Read the model definition and answer for the solid it produces. Units are mm, in the model's axes. Face numbers are marked on the shaded views. A direction names the side the tool comes from. Give positions to 0.01 mm unless a question says otherwise; leave off trailing zeros. Order: outer loops, then holes, each group sorted by start corner. A loop starts at its lowest first (then second) coordinate and runs counter-clockwise, first axis right, second up.
```python
from build123d import *

# Parameters (mm, degrees)
F0_R     = 6.375
F1_DEPTH = 8.26
F0_R_2   = 9.525
F2_DEPTH = 14.26
F3_W     = 13.49
F3_H     = 58.49083
F4_DEPTH = 38


with BuildPart() as f1:
    # F0 (on Front) → F1 (new body, symmetric)
    with BuildSketch(Plane.XZ):
        with BuildLine():
            Line((-26.615233, 45.963348), (-25.360972, 33.179498))
            ThreePointArc((-25.360972, 33.179498), (-9.404585, 28.615193), (4.051067, 38.330365))
            Line((4.051067, 38.330365), (10.939452, 38.330365))
            ThreePointArc((10.939452, 38.330365), (4.770442, 45.680142), (-0.28538, 53.835787))
            ThreePointArc((-0.28538, 53.835787), (-16.692609, 60.743646), (-26.615233, 45.963348))
        make_face()
        with Locations((-12.682133, 47.330365)):
            Circle(F0_R, mode=Mode.SUBTRACT)
    extrude(amount=F1_DEPTH, both=True)

    # F0 (on Front) → F2 (join, symmetric)
    with BuildSketch(Plane.XZ):
        with BuildLine():
            Line((-25.360972, 33.179498), (-21.894871, -2.14817))
            ThreePointArc((-21.894871, -2.14817), (-14.189314, -16.812596), (1.561379, -21.944523))
            Line((1.561379, -21.944523), (57, -18))
            Line((57, -18), (57, -6.375))
            Line((57, -6.375), (35, -6.375))
            ThreePointArc((35, -6.375), (28.625, 0), (35, 6.375))
            Line((35, 6.375), (57, 6.375))
            Line((57, 6.375), (57, 18))
            ThreePointArc((57, 18), (31.987423, 23.674071), (10.939452, 38.330365))
            Line((10.939452, 38.330365), (4.051067, 38.330365))
            ThreePointArc((4.051067, 38.330365), (-9.404585, 28.615193), (-25.360972, 33.179498))
        make_face()
        Circle(F0_R_2, mode=Mode.SUBTRACT)
    extrude(amount=F2_DEPTH, both=True)

    # F3 (on face) → F4 (cut)
    with BuildSketch(Plane.YZ.offset(57)):
        with Locations((0, -0.116389)):
            Rectangle(F3_W, F3_H)
    extrude(amount=-F4_DEPTH, mode=Mode.SUBTRACT)


solid = f1.part
```
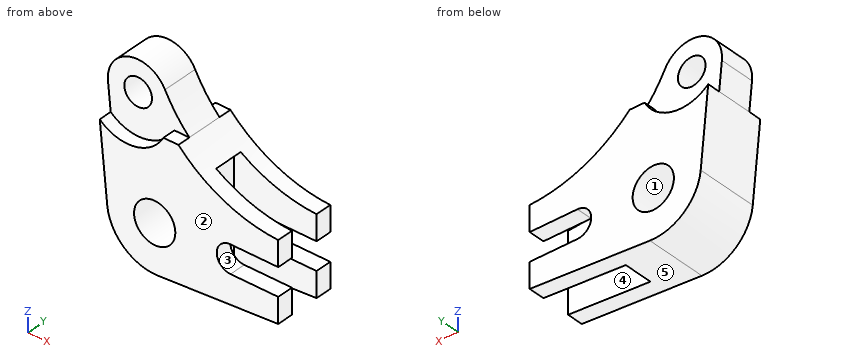
1) The part is cut by section D-D on z = 31.5. Determine the outline of the cut face in (x, y), and give its area (3 significant figures).
Final values:
outline: (-25.2, -14.26) - (-23.19, -14.26) - (-23.19, -8.26) - (-2.18, -8.26) - (-2.18, -14.26) - (18.67, -14.26) - (18.67, 14.26) - (-2.18, 14.26) - (-2.18, 8.26) - (-23.19, 8.26) - (-23.19, 14.26) - (-25.2, 14.26) - close
area: 999 mm2
2) A tool of negligible diameter and unlimited length cuts with its end or side. For the marked faces 4 and 5, from which of +Z, -Z, +X, -X, +Y, -Y can it reach the whole face along a straight path? Write none if from no direction.
Final values:
face 4: -Z, +X
face 5: -Z, +X, +Y, -Y
3) Consider L1, parallel to Y at x = 31.5, z = 6 (3 decimals); L2, parallel to Z at x = 0, y = -9.25 (3 decimals); L3, parallel to X at y = 10, z = 6.5. Determine where each line is inside the solid, lowest interval first.
Final values:
L1: y = -14.26 to -6.745, 6.745 to 14.26
L2: z = -22 to -9.525, 9.525 to 33.182
L3: x = -22.74 to -6.96, 6.96 to 57
4) Given pin 1 (6 mm diameter, centred on y = 4, z = 32, fed in from -X); pin 2 (8 mm diameter, centred on y = -10.5, z = 39, fed in from +X); pin 3 (5 mm diameter, centred on x = 7, y = -11, fed in from +Z), each flat-ended and moving along its own axis, determine where each tip first touches the part or whether it passes through.
Final values:
pin 1: stops at x = -25.54
pin 2: stops at x = 14.41
pin 3: stops at z = 38.33
5) The part is cut by section A-A on z = 0. Determine the outline of the cut face in (x, y) (3 decimals), and give its area (3 significant figures).
Final values:
outline: (-22.106, -14.26) - (-9.525, -14.26) - (-9.525, 14.26) - (-22.106, 14.26) - close; (9.525, -14.26) - (28.625, -14.26) - (28.625, -6.745) - (19, -6.745) - (19, 6.745) - (28.625, 6.745) - (28.625, 14.26) - (9.525, 14.26) - close
area: 774 mm2
6) The part is cut by section C-C on y = 2. Count the separate pieces of the cut face and the enclosed holes in it, and give its area (3 significant figures).
Final values:
separate pieces: 1
enclosed holes: 2
area: 2,610 mm2
7) The part is cut by section B-B on x = 51. Determine the outline of the cut face in (y, z) (3 decimals).
Final values:
outline: (-14.26, -18.427) - (-6.745, -18.427) - (-6.745, -6.375) - (-14.26, -6.375) - close; (-14.26, 6.375) - (-6.745, 6.375) - (-6.745, 18.453) - (-14.26, 18.453) - close; (6.745, -18.427) - (14.26, -18.427) - (14.26, -6.375) - (6.745, -6.375) - close; (6.745, 6.375) - (14.26, 6.375) - (14.26, 18.453) - (6.745, 18.453) - close
8) For a pull along X with two mould halves and no side action, classify the marked faces 1, 2 and 3 as released by +X, released by -X, zero draft, split by the parting line, or undercut.
Final values:
face 1: undercut
face 2: zero draft
face 3: released by +X
